from build123d import *

# Parameters (mm, degrees)
EXTRUDE_1_DEPTH = 2.5
SKETCH_2_R      = 0.3
EXTRUDE_2_DEPTH = 6
SKETCH_3_R      = 0.3
EXTRUDE_3_DEPTH = 3


with BuildPart() as part:
    # Эскиз1 → Бобышка-Вытянуть1 (new body)
    with BuildSketch(Plane(origin=(0, 0, 0), x_dir=(1, 0, 0), z_dir=(0, 1, 0))):
        Polygon((16.51, -0.526051224), (16.51, 0.526051224), (15.766051224, 1.27), (14.713948776, 1.27), (13.97, 0.526051224), (13.226051224, 1.27), (12.173948776, 1.27), (11.43, 0.526051224), (10.686051224, 1.27), (9.633948776, 1.27), (8.89, 0.526051224), (8.146051224, 1.27), (7.093948776, 1.27), (6.35, 0.526051224), (5.606051224, 1.27), (4.553948776, 1.27), (3.81, 0.526051224), (3.066051224, 1.27), (2.013948776, 1.27), (1.27, 0.526051224), (0.526051224, 1.27), (-0.526051224, 1.27), (-1.27, 0.526051224), (-1.27, -0.526051224), (-0.526051224, -1.27), (0.526051224, -1.27), (1.27, -0.526051224), (2.013948776, -1.27), (3.066051224, -1.27), (3.81, -0.526051224), (4.553948776, -1.27), (5.606051224, -1.27), (6.35, -0.526051224), (7.093948776, -1.27), (8.146051224, -1.27), (8.89, -0.526051224), (9.633948776, -1.27), (10.686051224, -1.27), (11.43, -0.526051224), (12.173948776, -1.27), (13.226051224, -1.27), (13.97, -0.526051224), (14.713948776, -1.27), (15.766051224, -1.27), align=None)
    extrude(amount=EXTRUDE_1_DEPTH)

    # Эскиз2 → Бобышка-Вытянуть2 (add)
    with BuildSketch(Plane(origin=(0, 2.5, 0), x_dir=(1, 0, 0), z_dir=(0, 1, 0))):
        Circle(SKETCH_2_R)
        with Locations((2.54, 0)):
            Circle(SKETCH_2_R)
        with Locations((5.08, 0)):
            Circle(SKETCH_2_R)
        with Locations((7.62, 0)):
            Circle(SKETCH_2_R)
        with Locations((10.16, 0)):
            Circle(SKETCH_2_R)
        with Locations((12.7, 0)):
            Circle(SKETCH_2_R)
        with Locations((15.24, 0)):
            Circle(SKETCH_2_R)
    extrude(amount=EXTRUDE_2_DEPTH)

    # Эскиз3 → Бобышка-Вытянуть3 (add)
    with BuildSketch(Plane.XZ):
        Circle(SKETCH_3_R)
        with Locations((2.54, 0)):
            Circle(SKETCH_3_R)
        with Locations((5.08, 0)):
            Circle(SKETCH_3_R)
        with Locations((7.62, 0)):
            Circle(SKETCH_3_R)
        with Locations((10.16, 0)):
            Circle(SKETCH_3_R)
        with Locations((12.7, 0)):
            Circle(SKETCH_3_R)
        with Locations((15.24, 0)):
            Circle(SKETCH_3_R)
    extrude(amount=EXTRUDE_3_DEPTH)


solid = part.part
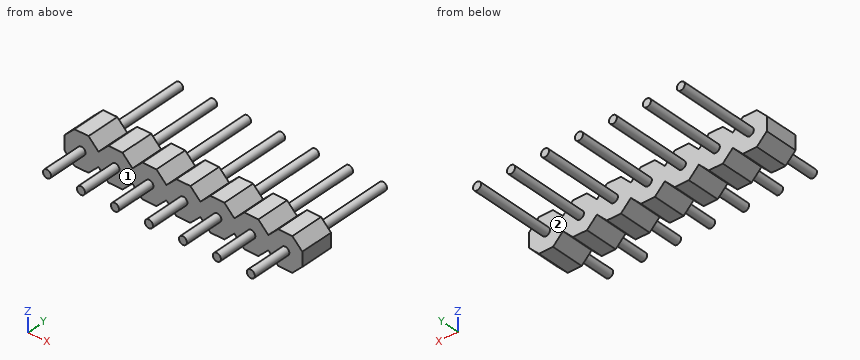
Design review of the part built by this model. Coordinates are the model's own, in mm. Face numbers are marked on the shaded views. Coordinates: 2 decimals unless noted, no trailing zeros. Order: outer loops, then holes, each group sorted by start corner. A loop starts at its lowest first (then second) coordinate and runs counter-clockwise, first axis right, second up. Notation, with made-up numbers: (27, 35) - (85, 35) arc R36 cw to (85, 73) - close; hole circle Ø1 at (40.25, -3). An arc over 180 degrees is marked (long way). Put each result on its own line as item: value.
1) Take a section at B-B, the plane x = 5.08. Give the boundary of the cut face in (y, z).
Response values:
outline: (-3, -0.3) - (0, -0.3) - (0, -1.27) - (2.5, -1.27) - (2.5, -0.3) - (8.5, -0.3) - (8.5, 0.3) - (2.5, 0.3) - (2.5, 1.27) - (0, 1.27) - (0, 0.3) - (-3, 0.3) - close
2) Take a section at C-C, the plane z = 0.95. Give the boundary of the cut face in (x, y).
Response values:
outline: (-0.85, 0) - (0.85, 0) - (0.85, 2.5) - (-0.85, 2.5) - close; (1.69, 0) - (3.39, 0) - (3.39, 2.5) - (1.69, 2.5) - close; (4.23, 0) - (5.93, 0) - (5.93, 2.5) - (4.23, 2.5) - close; (6.77, 0) - (8.47, 0) - (8.47, 2.5) - (6.77, 2.5) - close; (9.31, 0) - (11.01, 0) - (11.01, 2.5) - (9.31, 2.5) - close; (11.85, 0) - (13.55, 0) - (13.55, 2.5) - (11.85, 2.5) - close; (14.39, 0) - (16.09, 0) - (16.09, 2.5) - (14.39, 2.5) - close
3) Wall thickness on L1, parallel to Y at x = 0.25, z = -0.5; L2, parallel to Z at x = 2, y = 2; L3, parallel to Z at x = 12.5, y = -2: over which ranges is each line inside the solid? List them lowest first. Write a range as from..to.
Response values:
L1: y = 0..2.5
L2: z = -1.26..1.26
L3: z = -0.22..0.22
4) The part is to be moulded in two halves that separate along X. For the marked faces 1 and 2, say which applies: released by +X, released by -X, zero draft, split by the parting line, or undercut.
Response values:
face 1: undercut
face 2: undercut
5) Take a section at A-A, the plane y = -1.75. Give the boundary of the cut face in (x, z), and give its area (3 significant figures).
Response values:
outline: circle Ø0.6 at (0, 0); circle Ø0.6 at (2.54, 0); circle Ø0.6 at (5.08, 0); circle Ø0.6 at (7.62, 0); circle Ø0.6 at (10.16, 0); circle Ø0.6 at (12.7, 0); circle Ø0.6 at (15.24, 0)
area: 1.98 mm²
6) Insertion check: P1, Ø1, axis at x = 10, y = -1.5, coming from the +Z side. The pin has a flat end and moves straight along its axis. Give the tip position at first contact, or say it passes through.
Response values:
P1: stops at z = 0.3
7) Take a section at D-D, the plane x = 10.25. Give the boundary of the cut face in (y, z), and give its area (3 significant figures).
Response values:
outline: (-3, -0.29) - (0, -0.29) - (0, -1.27) - (2.5, -1.27) - (2.5, -0.29) - (8.5, -0.29) - (8.5, 0.29) - (2.5, 0.29) - (2.5, 1.27) - (0, 1.27) - (0, 0.29) - (-3, 0.29) - close
area: 11.5 mm²
